For this review, take the finished solid that the model builds, in its own axes (mm). A direction names the side the tool comes from. Coordinates: 2 decimals unless noted, no trailing zeros. Write each loop counter-clockwise with the first axis right and the second up, starting at its lowest first coordinate (ties: lowest second). Pieces come first, ordered by that corner, then holes.
```python
from build123d import *

# Parameters (mm, degrees)
F1_DEPTH = 12.7
F2_DEPTH = 44.45
F0_W     = 31.75
F0_H     = 8.428902
F3_DEPTH = 44.45
F4_R     = 6.35
F5_DEPTH = 14.224


with BuildPart() as f1:
    # F0 (on Top) → F1 (new body)
    with BuildSketch(Plane.XY):
        Polygon((-62.563881, 0), (-61.939803, 0), (-32.672367, 0), (-32.672367, 12.7), (-13.622367, 31.75), (11.777633, 31.75), (30.827633, 12.7), (30.827633, 0), (65.060197, 0), (65.060197, 22.098), (13.183661, 69.596), (13.183661, 61.167098), (-18.566339, 61.167098), (-18.566339, 69.596), (-62.563881, 22.098), align=None)
    extrude(amount=F1_DEPTH)

    # F0 (on Top) → F2 (join)
    with BuildSketch(Plane.XY):
        Polygon((-32.672367, 12.7), (-32.672367, 0), (30.827633, 0), (30.827633, 12.7), (11.777633, 31.75), (-13.622367, 31.75), align=None)
    extrude(amount=F2_DEPTH)

    # F0 (on Top) → F3 (join)
    with BuildSketch(Plane.XY):
        with Locations((-2.691339, 65.381549)):
            Rectangle(F0_W, F0_H)
    extrude(amount=F3_DEPTH)

    # F4 (on face) → F5 (cut)
    with BuildSketch(Plane(origin=(0, 69.596, 0), x_dir=(-1, 0, 0), z_dir=(0, 1, 0))):
        with Locations((2.691339, 28.702)):
            Circle(F4_R)
    extrude(amount=-F5_DEPTH, mode=Mode.SUBTRACT)


solid = f1.part
```
1) The part is to be moulded in two halves that separate along Y. For faces 1 (the face through (-3, 69.596, 22)), 2 (the face through (65.06, 11, 6)), 3 (the face through (-1, 31.75, 28)), say which applies: pulls with the +Y half, pulls with the -Y half, needs draft (parallel to the pull), parting line crosses it, or undercut.
2) Consider section D-D (z = 30). Give the boundary of the cut face in (x, y), then the cut area to 3 significant figures.
3) Consider section B-B (y = 11). Give the boundary of the cut face in (x, z), then the cut area to 3 significant figures.
4) Clearance check with flat-ended pins moving along their axes: P1, Ø6.5, axis at y = 64, z = 23.5, coming from the -X side; P2, Ø10, axis at y = 55, z = 6, coming from the -X side; P3, Ø1.5, axis at y = 41, z = 10, coming from the +X side. State where each tip first meets the part, or that it passes through.
5) For L1, parallel to Y at x = 8, z = 39; L2, parallel to Z at x = 29, y = 32; L3, parallel to X at y = 9, z = 32.5, list the stretches that pass through material, from the lowest coordinate up.
6) Consider section C-C (x = 9.5). Give the boundary of the cut face in (y, z).
7) Consider section A-A (z = 36.5). Give the boundary of the cut face in (x, y).
8) Tool access review of faces 4 (the face through (13.184, 65, 28)), 5 (the face through (-32.672, 6, 28)), 6 (the face through (-1.865, 65.441, 34.998)), 7 (the face through (-23.01, 22.36, 28.35)): name each direction out of +Z, -Z, +X, -X, +Y, -Y from which nothing blocks a thin tool from reaching the whole face with its end or side.
Results:
1. face 1: pulls with the +Y half
1. face 2: needs draft
1. face 3: undercut
2. outline: (-32.67, 0) - (30.83, 0) - (30.83, 12.7) - (11.78, 31.75) - (-13.62, 31.75) - (-32.67, 12.7) - close; (-18.57, 61.17) - (-8.91, 61.17) - (-8.91, 69.6) - (-18.57, 69.6) - close; (3.52, 61.17) - (13.18, 61.17) - (13.18, 69.6) - (3.52, 69.6) - close
2. area: 1,820 mm2
3. outline: (-62.56, 0) - (65.06, 0) - (65.06, 12.7) - (30.83, 12.7) - (30.83, 44.45) - (-32.67, 44.45) - (-32.67, 12.7) - (-62.56, 12.7) - close
3. area: 3,640 mm2
4. P1: stops at x = -18.57
4. P2: stops at x = -36.72
4. P3: stops at x = 45.23
5. L1: y = 0 to 31.75, 61.17 to 69.6
5. L2: z = 0 to 12.7
5. L3: x = -32.67 to 30.83
6. outline: (0, 0) - (69.6, 0) - (69.6, 44.45) - (61.17, 44.45) - (61.17, 12.7) - (31.75, 12.7) - (31.75, 44.45) - (0, 44.45) - close
7. outline: (-32.67, 0) - (30.83, 0) - (30.83, 12.7) - (11.78, 31.75) - (-13.62, 31.75) - (-32.67, 12.7) - close; (-18.57, 61.17) - (13.18, 61.17) - (13.18, 69.6) - (-18.57, 69.6) - close
8. face 4: +Z, +X, +Y
8. face 5: +Z, -X, +Y, -Y
8. face 6: +Y
8. face 7: +Z, -X
